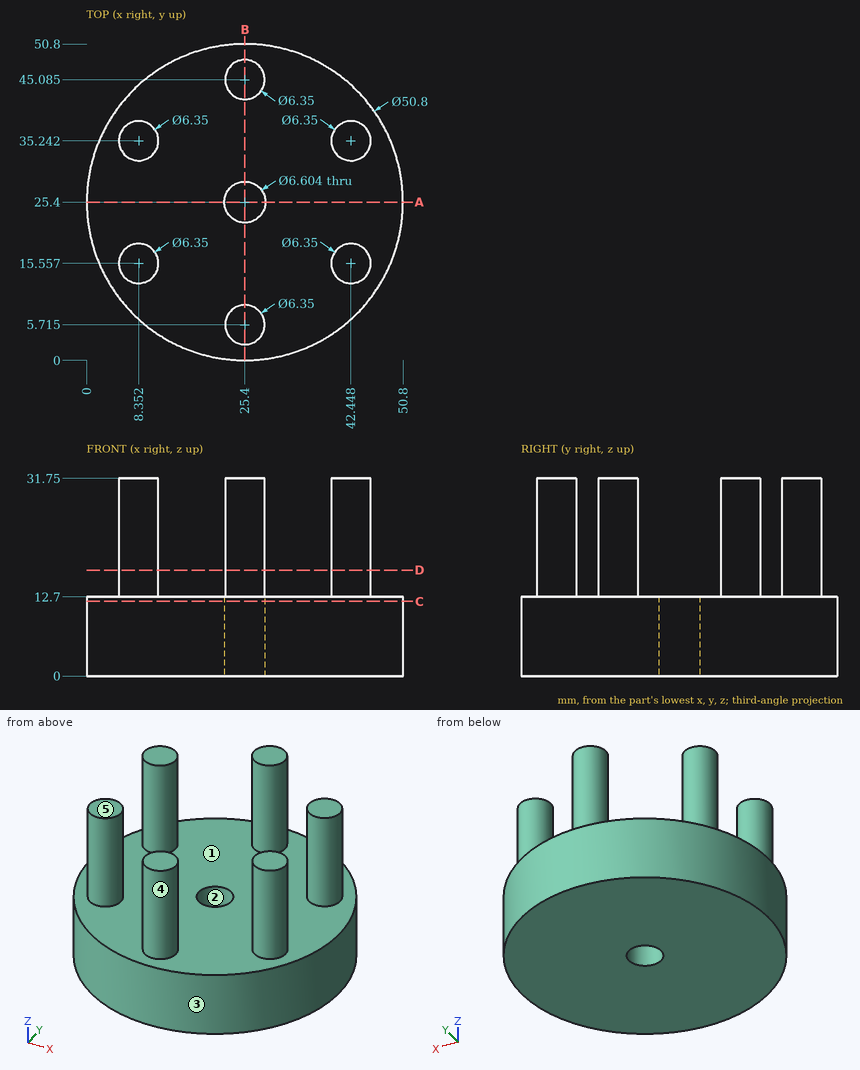
Source: three-view drawing plus pictorial views. Frame: mm from the lowest corner of the part. A direction names the side the tool comes from. Coordinates: 2 decimals unless noted, no trailing zeros. Write each loop counter-clockwise with the first axis right and the second up, starting at its lowest first coordinate (ties: lowest second). Pieces come first, ordered by that corner, then holes. Notation, with made-up numbers: (-38.5, -33) -> (-1.5, -33) arc R21 ccw to (-1.5, -8) -> close; hole circle Ø5 at (59.5, 78). An arc over 180 degrees is marked (long way). Write each question's results on one line, items separated by ' | '.
Item 1: Material intervals for probe 1 along Y at (x, z) = (25.4, 3.25); probe 2 along Z at (x, y) = (10, 11); probe 3 along Y at (x, z) = (41, 22) (1 decimal), sorted ascending.
Conclusion:
probe 1: y = 0 to 22.1, 28.7 to 50.8 | probe 2: z = 0 to 12.7 | probe 3: y = 12.7 to 18.4, 32.4 to 38.1
Item 2: Pin query (flat end, axial travel): pin 1 Ø4 at (x, z) = (31, 12) entering from +Y; pin 2 Ø5 at (x, y) = (38, 5.5) entering from +Z; pin 3 Ø3 at (y, z) = (42.5, 25.5) entering from -X. Return the tip coordinate at first contact, or that it passes through.
Conclusion:
pin 1: stops at y = 50.54 | pin 2: stops at z = 12.7 | pin 3: stops at x = 22.42
Item 3: Section query B-B on x = 25.4. Return loops of the section in (y, z).
Conclusion:
outline: (0, 0) -> (22.1, 0) -> (22.1, 12.7) -> (8.89, 12.7) -> (8.89, 31.75) -> (2.54, 31.75) -> (2.54, 12.7) -> (0, 12.7) -> close; (28.7, 0) -> (50.8, 0) -> (50.8, 12.7) -> (48.26, 12.7) -> (48.26, 31.75) -> (41.91, 31.75) -> (41.91, 12.7) -> (28.7, 12.7) -> close
Item 4: Set-up query: the marked faces 1 and 2. Return all of +Z, -Z, +X, -X, +Y, -Y with unobstructed straight access to the full face (end or side cutting, diameter ignored); none if empty.
Conclusion:
face 1: +Z | face 2: +Z, -Z
Item 5: Section query A-A on y = 25.4. Return loops of the section in (x, z).
Conclusion:
outline: (0, 0) -> (22.1, 0) -> (22.1, 12.7) -> (0, 12.7) -> close; (28.7, 0) -> (50.8, 0) -> (50.8, 12.7) -> (28.7, 12.7) -> close
Item 6: Section query C-C on z = 12. Return loops of the section in (x, y) (1 decimal).
Conclusion:
outline: circle Ø50.8 at (25.4, 25.4); hole circle Ø6.6 at (25.4, 25.4)
Item 7: Section query D-D on z = 17. Count the separate pieces of the cut face and the enclosed holes in it, plus the area to 3 significant figures.
Conclusion:
separate pieces: 6 | enclosed holes: 0 | area: 190 mm^2
Item 8: Mould query, pull axis Y, two halves, no side actions, for the marked faces 3, 4 and 5. Classes: +Y half, -Y half, draft (parallel to the pull), parting line (faces both ways), or undercut.
Conclusion:
face 3: parting line | face 4: undercut | face 5: draft
